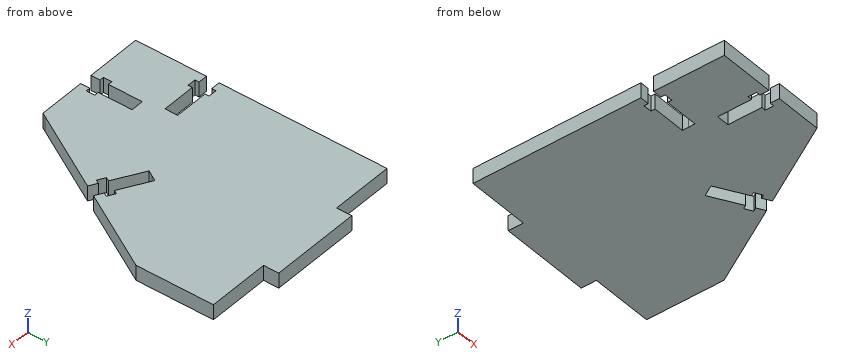
```python
from build123d import *

# Parameters (mm, degrees)
BOSS_EXTRUDE1_DEPTH = 5
CUT_EXTRUDE3_START  = -5
CUT_EXTRUDE3_DEPTH  = 5
BOSS_EXTRUDE2_DEPTH = 5


# Read off the part's stored shape, not the designer's step: Cut-Extrude3
with BuildPart() as part:
    # Sketch1 → Boss-Extrude1 (new body)
    with BuildSketch(Plane.XY):
        Polygon((-35.261138019, -40.918717749), (2.830677256, -40.918717749), (3.530317734, -39.706904894), (36.028317734, 16.581282251), (36.028317734, 42.200866684), (-35.231632156, 42.261282251), align=None)
    extrude(amount=BOSS_EXTRUDE1_DEPTH)

    # Cut-Extrude3 outline → Cut-Extrude3 (cut)
    with BuildSketch(Plane.XY.offset(5).offset(CUT_EXTRUDE3_START)):
        Polygon((16.125363943, -11.891644937), (18.722168425, -13.393847636), (20.82216918, -9.756539633), (18.228446966, -8.256119968), (18.930502063, -7.044872657), (16.506818751, -5.642817308), (15.805791076, -6.854658964), (6.110026049, -1.245840704), (5.056943403, -3.062711671), (4.006943025, -4.881365673), (13.702708053, -10.490183932), (13.001680379, -11.702025589), (15.425363691, -13.104080938), align=None)
        Polygon((-35.251344401, -13.309523063), (-35.25283547, -17.512996385), (-32.25134298, -17.512996385), (-32.2508476, -18.909523063), (-29.4508476, -18.909523063), (-29.4508476, -17.509523063), (-18.251343332, -17.509523063), (-18.25208825, -15.409523063), (-18.251343332, -13.309523063), (-29.4508476, -13.309523063), (-29.4508476, -11.909523063), (-32.2508476, -11.909523063), (-32.251344213, -13.309523063), align=None)
        Polygon((-16.848777516, -40.918717749), (-12.648777516, -40.918717749), (-12.648777516, -37.918717749), (-11.248777516, -37.918717749), (-11.248777516, -35.118717749), (-12.648777516, -35.118717749), (-12.648777516, -23.918717749), (-16.848777516, -23.918717749), (-16.848777516, -35.118717749), (-18.248777516, -35.118717749), (-18.248777516, -37.918717749), (-16.848777516, -37.918717749), align=None)
    extrude(amount=CUT_EXTRUDE3_DEPTH, mode=Mode.SUBTRACT)

    # Sketch3 → Boss-Extrude2 (add)
    with BuildSketch(Plane.XY.offset(5)):
        Polygon((-14.56360213, 47.243759494), (15.43639787, 47.243759494), (15.43639787, 42.218324913), (-14.56360213, 42.243759494), align=None)
    extrude(amount=-BOSS_EXTRUDE2_DEPTH)


solid = part.part
```
Could you check a few things on this model? Use its own coordinates, in mm. Give positions to 0.01 mm unless a question says otherwise; leave off trailing zeros. Loops run counter-clockwise (first coordinate to the right, second up) from the corner with the lowest first, then second, coordinate; pieces in that order, holes last. Notation, with made-up numbers: (-7, -13) - (1, -13) arc R21 cw to (1, -1) - close; hole circle Ø5 at (60.5, -15.5). An arc over 180 degrees is marked (long way). Use one line per item in the form item = value.
1. I want a section at D-D (y = -14.5). Please give me the cut outline in (x, z).
Response values:
outline = (-18.25, 0) - (18.08, 0) - (18.08, 5) - (-18.25, 5) - close
2. I'm going to push flat-ended pins straight in: pin 1 Ø1.5 at (y, z) = (-26.5, 1.5) entering from -X; pin 2 Ø1.5 at (x, z) = (-25, 2) entering from +Y; pin 3 Ø1.5 at (y, z) = (45, 1.5) entering from +X. Where does each tip first touch, or does it pass through?
Response values:
pin_1 = -35.26
pin_2 = 42.25
pin_3 = 15.44
3. I want a section at A-A (x = 8.5). Please give me the cut outline in (y, z), and give its area (3 significant figures).
Response values:
outline = (-31.1, 0) - (-7.48, 0) - (-7.48, 5) - (-31.1, 5) - close; (-2.63, 0) - (47.24, 0) - (47.24, 5) - (-2.63, 5) - close
area = 367 mm²
4. I need wall thicknesses on probe 1 along Y at (x, z) = (-21.5, 2.05); probe 2 along Y at (x, z) = (-13, 4). Which ranges of each line are inside material? Lowest first, please.
Response values:
probe_1 = -40.92 to -17.51, -13.31 to 42.25
probe_2 = -23.92 to 47.24
5. I want a section at C-C (x = 30). Please give me the cut outline in (y, z).
Response values:
outline = (6.14, 0) - (42.21, 0) - (42.21, 5) - (6.14, 5) - close
6. I want a section at B-B (y = -30). Please give me the cut outline in (x, z).
Response values:
outline = (-35.26, 0) - (-16.85, 0) - (-16.85, 5) - (-35.26, 5) - close; (-12.65, 0) - (9.13, 0) - (9.13, 5) - (-12.65, 5) - close
